```python
from build123d import *

# Parameters (mm, degrees)
F1_DEPTH  = 3.5
F2_DEPTH  = 11
F4_DEPTH  = 25
F5_W      = 2.5
F5_H      = 10
F6_DEPTH  = 42.5
F7_W      = 2.5
F7_H      = 10
F7_W_2    = 6
F8_DEPTH  = 2.5
F9_R      = 2
F10_R     = 5
F11_R     = 2.75
F12_DEPTH = 3.2


# Not quite as in the source:
# - a pattern or mirror of a feature is missing from the dataset's text; its kind, count and spacing are read off the source's solid


with BuildPart() as f1:
    # F0 (on Top) → F1 (new body)
    with BuildSketch(Plane.XY):
        with BuildLine():
            ThreePointArc((25.385, 17.035), (22.9393416229, 22.9393416229), (17.035, 25.385))
            Line((17.035, 25.385), (-17.035, 25.385))
            ThreePointArc((-17.035, 25.385), (-22.9393416229, 22.9393416229), (-25.385, 17.035))
            Line((-25.385, 17.035), (-25.385, -17.035))
            ThreePointArc((-25.385, -17.035), (-22.9393416229, -22.9393416229), (-17.035, -25.385))
            Line((-17.035, -25.385), (17.035, -25.385))
            ThreePointArc((17.035, -25.385), (22.9393416229, -22.9393416229), (25.385, -17.035))
            Line((25.385, -17.035), (25.385, 17.035))
        make_face()
    extrude(amount=F1_DEPTH)

    # F0 (on Top) → F2 (join)
    with BuildSketch(Plane.XY):
        with BuildLine():
            ThreePointArc((27.885, 17.035), (24.7071085759, 24.7071085759), (17.035, 27.885))
            Line((17.035, 27.885), (-17.035, 27.885))
            ThreePointArc((-17.035, 27.885), (-24.7071085759, 24.7071085759), (-27.885, 17.035))
            Line((-27.885, 17.035), (-27.885, -17.035))
            ThreePointArc((-27.885, -17.035), (-24.7071085759, -24.7071085759), (-17.035, -27.885))
            Line((-17.035, -27.885), (17.035, -27.885))
            ThreePointArc((17.035, -27.885), (24.7071085759, -24.7071085759), (27.885, -17.035))
            Line((27.885, -17.035), (27.885, 17.035))
        make_face()
        with BuildLine():
            Line((-17.035, 25.385), (17.035, 25.385))
            ThreePointArc((17.035, 25.385), (22.9393416229, 22.9393416229), (25.385, 17.035))
            Line((25.385, 17.035), (25.385, -17.035))
            ThreePointArc((25.385, -17.035), (22.9393416229, -22.9393416229), (17.035, -25.385))
            Line((17.035, -25.385), (-17.035, -25.385))
            ThreePointArc((-17.035, -25.385), (-22.9393416229, -22.9393416229), (-25.385, -17.035))
            Line((-25.385, -17.035), (-25.385, 17.035))
            ThreePointArc((-25.385, 17.035), (-22.9393416229, 22.9393416229), (-17.035, 25.385))
        make_face(mode=Mode.SUBTRACT)
    extrude(amount=F2_DEPTH)

    # F3 (on face) → F4 (cut)
    with BuildSketch(Plane.XZ.offset(27.885)):
        with BuildLine():
            ThreePointArc((-9.4494897428, 11), (-8.9364916731, 8.9188611699), (-7, 8))
            Line((-7, 8), (7, 8))
            ThreePointArc((7, 8), (8.9364916731, 8.9188611699), (9.4494897428, 11))
            Line((9.4494897428, 11), (-9.4494897428, 11))
        make_face()
        with BuildLine():
            ThreePointArc((-7, 13), (-8.5811388301, 12.4364916731), (-9.4494897428, 11))
            Line((-9.4494897428, 11), (9.4494897428, 11))
            ThreePointArc((9.4494897428, 11), (8.5811388301, 12.4364916731), (7, 13))
            Line((7, 13), (-7, 13))
        make_face()
    extrude(amount=-F4_DEPTH, mode=Mode.SUBTRACT)

    # F5 (on face) → F6 (join)
    with BuildSketch(Plane.XY.offset(11)):
        with Locations((26.635, 0)):
            Rectangle(F5_W, F5_H)
    f6 = extrude(amount=F6_DEPTH)

    # F6_copies: F6 across plane
    add(f6.mirror(Plane(origin=(0, 0, 0), x_dir=(0, 0, -1), z_dir=(-1, 0, 0))))

    # F7 (on face) → F8 (join)
    with BuildSketch(Plane.XY.offset(53.5)):
        with Locations((26.635, 0)):
            Rectangle(F7_W, F7_H)
        with Locations((22.385, 0)):
            Rectangle(F7_W_2, F7_H)
    f8 = extrude(amount=F8_DEPTH)

    # F8_copies: F8 across plane
    add(f8.mirror(Plane(origin=(0, 0, 0), x_dir=(0, 0, -1), z_dir=(-1, 0, 0))))

    # F9
    f9_edges = [f1.edges().sort_by_distance(p)[0] for p in [
        (25.385, 0, 53.5),
        (27.885, 0, 56),
        (-25.385, 0, 53.5),
        (-27.885, 0, 56),
    ]]
    fillet(f9_edges, radius=F9_R)

    # F10
    f10_edges = [f1.edges().sort_by_distance(p)[0] for p in [
        (26.635, 5, 11),
        (26.635, -5, 11),
        (-26.635, 5, 11),
        (-26.635, -5, 11),
    ]]
    fillet(f10_edges, radius=F10_R)

    # F11 (on face) → F12 (cut)
    with BuildSketch(Plane.XY.offset(3.5)):
        with Locations((0, -15)):
            Circle(F11_R)
        with Locations((14.2658477444, -4.6352549156)):
            Circle(F11_R)
        with Locations((8.8167787844, 12.1352549156)):
            Circle(F11_R)
        with Locations((-8.8167787844, 12.1352549156)):
            Circle(F11_R)
        with Locations((-14.2658477444, -4.6352549156)):
            Circle(F11_R)
    extrude(amount=-F12_DEPTH, mode=Mode.SUBTRACT)


solid = f1.part
```
Could you check a few things on this model? Use its own coordinates, in mm. A direction names the side the tool comes from. Round coordinates to 2 decimals unless told otherwise and drop trailing zeros. Write each loop counter-clockwise with the first axis right and the second up, starting at its lowest first coordinate (ties: lowest second). Pieces come first, ordered by that corner, then holes. Notation, with made-up numbers: M -25,-17 L -7,-17 A23 cw -7,1 Z; hole C -37.5,76.5 d1. An arc over 180 degrees is marked long. Write each question's results on one line, items separated by ' | '. Start each with the question number.
1. I'm going to push flat-ended pins straight in: pin 1 Ø9 at (x, y) = (-8.82, 12.14) entering from +Z; pin 2 Ø7 at (x, z) = (22, 44) entering from -Y; pin 3 Ø2 at (x, y) = (1.5, -26.5) entering from +Z. Where does each tip first touch, or does it pass through?
2. On a 3-axis mill with a long thin cutter (end or side, diameter ignored), from which of +Z, -Z, +X, -X, +Y, -Y can I reach the whole of each face in a straight line? I mean faces 1 (the face through (26, 5, 39)), 2 (the face through (-7.338, 14.454, 1.922)), 3 (the face through (21, 0, 53.5)), 4 (the face through (26, -5, 39)). Say none if no direction works.
3. I need wall thicknesses on L1, parallel to X at y = -0.5, z = 28.5 (3 decimals); L2, parallel to Y at x = 0, z = 1 (3 decimals); L3, parallel to Z at x = 25, y = 22. Which ranges of each line are inside material? Lowest first, please. Write a range as from..to.
4. Thinking about a two-plate mould opening in Y: for faces 5 (the face through (0, 25.385, 7)), 6 (the face through (-26, 5, 39)), 7 (the face through (-0.358, -12.273, 1.922)), 8 (the face through (-27.315, 0.07, 55.399)), which applies, +Y half, -Y half, draft (parallel to the pull), parting line (faces both ways), or undercut?
5. Imagine slicing it at A-A on y = -15. List the corners of the cut face in (x, z) for me (3 decimals).
6. Imagine slicing it at C-C on x = -4. List the corners of the cut face in (y, z) for me (3 decimals), and give its area (3 significant figures).
7. Imagine slicing it at D-D on x = -21. List the corners of the cut face in (y, z) for me, and give its area (3 significant figures).
8. Imagine slicing it at B-B on z = 24. List the corners of the cut face in (x, y) for me (3 decimals).
Result sheet:
1) pin 1: stops at z = 3.5 | pin 2: stops at y = -5 | pin 3: stops at z = 8
2) face 1: +Z, +X, -X, +Y | face 2: +Z | face 3: +Y, -Y | face 4: +Z, +X, -X, -Y
3) L1: x = -27.885..-25.385, 25.385..27.885 | L2: y = -27.885..-17.75, -12.25..27.885 | L3: z = 0..11
4) face 5: undercut | face 6: +Y half | face 7: undercut | face 8: draft
5) outline: M -27.885,0 L 27.885,0 L 27.885,11 L 25.385,11 L 25.385,3.5 L 2.75,3.5 L 2.75,0.3 L -2.75,0.3 L -2.75,3.5 L -25.385,3.5 L -25.385,11 L -27.885,11 Z
6) outline: M -27.885,0 L 27.885,0 L 27.885,11 L 25.385,11 L 25.385,3.5 L -25.385,3.5 L -25.385,8 L -27.885,8 Z | area: 225 mm^2
7) outline: M -27.13,0 L 27.13,0 L 27.13,11 L 24.38,11 L 24.38,3.5 L -24.38,3.5 L -24.38,11 L -27.13,11 Z; M -5,53.5 L 5,53.5 L 5,56 L -5,56 Z | area: 256 mm^2
8) outline: M -27.885,-5 L -25.385,-5 L -25.385,5 L -27.885,5 Z; M 25.385,-5 L 27.885,-5 L 27.885,5 L 25.385,5 Z
